from build123d import *

# Parameters (mm, degrees)
CROQUIS1_R              = 2
CROQUIS1_R_2            = 1.5
CROQUIS1_W              = 3
CROQUIS1_H              = 10
SALIENTE_EXTRUIR1_DEPTH = 3


with BuildPart() as part:
    # Croquis1 → Saliente-Extruir1 (new body)
    with BuildSketch(Plane(origin=(0, 0, 0), x_dir=(1, 0, 0), z_dir=(0, 1, 0))):
        with BuildLine():
            Line((-30, -21.975186569), (-30, 62.5))
            Line((-30, 62.5), (-4.123983247, 62.5))
            Line((-4.123983247, 62.5), (-4.123983247, 59.5))
            Line((-4.123983247, 59.5), (5.876016753, 59.5))
            Line((5.876016753, 59.5), (5.876016753, 62.5))
            Line((5.876016753, 62.5), (30, 62.5))
            Line((30, 62.5), (30, -21.975186569))
            Line((30, -21.975186569), (30, -31))
            ThreePointArc((30, -31), (31.171572875, -33.828427125), (34, -35))
            Line((34, -35), (50.699653605, -35))
            ThreePointArc((50.699653605, -35), (55.61862518, -37.564345966), (56.332948449, -43.06542712))
            ThreePointArc((56.332948449, -43.06542712), (44.677053609, -62.460636323), (26.666666667, -76.159540905))
            ThreePointArc((26.666666667, -76.159540905), (20.83772234, -75.883721919), (18, -70.784702406))
            Line((18, -70.784702406), (18, -67.5))
            ThreePointArc((18, -67.5), (16.828427125, -64.671572875), (14, -63.5))
            Line((14, -63.5), (12, -63.5))
            ThreePointArc((12, -63.5), (9.171572875, -64.671572875), (8, -67.5))
            Line((8, -67.5), (8, -80))
            ThreePointArc((8, -80), (0, -88), (-8, -80))
            Line((-8, -80), (-8, -67.5))
            ThreePointArc((-8, -67.5), (-9.171572875, -64.671572875), (-12, -63.5))
            Line((-12, -63.5), (-14, -63.5))
            ThreePointArc((-14, -63.5), (-16.828427125, -64.671572875), (-18, -67.5))
            Line((-18, -67.5), (-18, -70.784702406))
            ThreePointArc((-18, -70.784702406), (-20.83772234, -75.883721919), (-26.666666667, -76.159540905))
            ThreePointArc((-26.666666667, -76.159540905), (-44.677053609, -62.460636323), (-56.332948449, -43.06542712))
            ThreePointArc((-56.332948449, -43.06542712), (-55.61862518, -37.564345966), (-50.699653605, -35))
            Line((-50.699653605, -35), (-34, -35))
            ThreePointArc((-34, -35), (-31.171572875, -33.828427125), (-30, -31))
            Line((-30, -31), (-30, -21.975186569))
        make_face()
        with Locations(Location((-24.3, 37.439181633, 0), (0, 0, 270))):
            Circle(CROQUIS1_R, mode=Mode.SUBTRACT)
        with Locations(Location((16.54, 52.26006939, 0), (0, 0, 270))):
            Circle(CROQUIS1_R_2, mode=Mode.SUBTRACT)
        with Locations(Location((16.54, 34.48006939, 0), (0, 0, 270))):
            Circle(CROQUIS1_R_2, mode=Mode.SUBTRACT)
        with Locations(Location((-16.48, 34.48006939, 0), (0, 0, 270))):
            Circle(CROQUIS1_R_2, mode=Mode.SUBTRACT)
        with Locations(Location((-16.48, 52.26006939, 0), (0, 0, 270))):
            Circle(CROQUIS1_R_2, mode=Mode.SUBTRACT)
        with Locations((28.5, -55)):
            Rectangle(CROQUIS1_W, CROQUIS1_H, mode=Mode.SUBTRACT)
        with Locations((-28.5, -55)):
            Rectangle(CROQUIS1_W, CROQUIS1_H, mode=Mode.SUBTRACT)
        with BuildLine():
            Line((1.5, -65), (1.5, -80))
            ThreePointArc((1.5, -80), (0, -81.5), (-1.5, -80))
            Line((-1.5, -80), (-1.5, -65))
            ThreePointArc((-1.5, -65), (0, -63.5), (1.5, -65))
        make_face(mode=Mode.SUBTRACT)
        with BuildLine():
            Line((7.5, -20), (-7.5, -20))
            ThreePointArc((-7.5, -20), (-11.035533906, -18.535533906), (-12.5, -15))
            Line((-12.5, -15), (-12.5, 15))
            ThreePointArc((-12.5, 15), (-11.035533906, 18.535533906), (-7.5, 20))
            Line((-7.5, 20), (7.5, 20))
            ThreePointArc((7.5, 20), (11.035533906, 18.535533906), (12.5, 15))
            Line((12.5, 15), (12.5, -15))
            ThreePointArc((12.5, -15), (11.035533906, -18.535533906), (7.5, -20))
        make_face(mode=Mode.SUBTRACT)
        with BuildLine():
            ThreePointArc((-52.107977316, -41.51635678), (-41.326274588, -59.456925292), (-24.666666667, -72.12841203))
            ThreePointArc((-24.666666667, -72.12841203), (-22.656290375, -71.451369072), (-23.333333333, -69.440992781))
            ThreePointArc((-23.333333333, -69.440992781), (-39.092421908, -57.454451272), (-49.291329893, -40.48364322))
            ThreePointArc((-49.291329893, -40.48364322), (-51.216010385, -39.591676289), (-52.107977316, -41.51635678))
        make_face(mode=Mode.SUBTRACT)
        with BuildLine():
            ThreePointArc((52.107977316, -41.51635678), (41.326274588, -59.456925292), (24.666666667, -72.12841203))
            ThreePointArc((24.666666667, -72.12841203), (22.656290375, -71.451369072), (23.333333333, -69.440992781))
            ThreePointArc((23.333333333, -69.440992781), (39.092421908, -57.454451272), (49.291329893, -40.48364322))
            ThreePointArc((49.291329893, -40.48364322), (51.216010385, -39.591676289), (52.107977316, -41.51635678))
        make_face(mode=Mode.SUBTRACT)
    extrude(amount=SALIENTE_EXTRUIR1_DEPTH)


solid = part.part
Geometry: final body of the model. Coordinates: model frame, mm. A direction names the side the tool comes from. Coordinates: 2 decimals unless noted, no trailing zeros. Order: outer loops, then holes, each group sorted by start corner. A loop starts at its lowest first (then second) coordinate and runs counter-clockwise, first axis right, second up.
1) Section A-A (x = -44.5). Return loops of the section in (y, z).
Result sheet:
outline: (0, 35) - (3, 35) - (3, 50.27) - (0, 50.27) - close; (0, 55.58) - (3, 55.58) - (3, 62.66) - (0, 62.66) - close
2) Section D-D (x = 36.5). Return loops of the section in (y, z), then the cut area to 3 significant figures.
Result sheet:
outline: (0, 35) - (3, 35) - (3, 60.15) - (0, 60.15) - close; (0, 64.22) - (3, 64.22) - (3, 70.03) - (0, 70.03) - close
area: 92.9 mm2
3) Set-up query: faces 4 (the flat face through (27, 1, 55)), 5 (the flat face through (30, 1, -16)), 6 (the flat face through (1, 1, -59.5)), 7 (the cylindrical face through (16.859, 1.479, 64.703)). Return all of +Z, -Z, +X, -X, +Y, -Y with unobstructed straight access to the full face (end or side cutting, diameter ignored); none if empty.
Result sheet:
face 4: +Y, -Y
face 5: -Z, +X, +Y, -Y
face 6: -Z, +Y, -Y
face 7: +Z, +Y, -Y
4) Ray query, probe 1 along X at (y, z) = (2.45, -2.5); probe 2 along X at (y, z) = (1.05, 57); probe 3 along X at (y, z) = (2.2, 70). Return the intervals inside material, ascending.
Result sheet:
probe 1: x = -30 to -12.5, 12.5 to 30
probe 2: x = -49.03 to -43.4, -39.5 to -30, -27 to 27, 30 to 39.5, 43.4 to 49.03
probe 3: x = -36.54 to -28.56, -22.72 to -18, -8 to -1.5, 1.5 to 8, 18 to 22.72, 28.56 to 36.54
5) Section B-B (z = 74). Return loops of the section in (x, y).
Result sheet:
outline: (-30.64, 0) - (-18.93, 0) - (-18.93, 3) - (-30.64, 3) - close; (-8, 0) - (-1.5, 0) - (-1.5, 3) - (-8, 3) - close; (1.5, 0) - (8, 0) - (8, 3) - (1.5, 3) - close; (18.93, 0) - (30.64, 0) - (30.64, 3) - (18.93, 3) - close
6) Section C-C (y = 0.75). Give the number of separate pieces and of enclosed holes in the cut face, then the cut area to 3 significant figures.
Result sheet:
separate pieces: 1
enclosed holes: 11
area: 8,250 mm2
7) Draft query along Z for faces 1 (the cylindrical face through (-44.46, 1.48, 62.7)), 2 (the flat face through (-4.124, 1, -61)), 3 (the cylindrical face through (-17.81, 1.48, -51.57)). Return one class per face: released by +Z, released by -Z, zero draft, split by the parting line, or undercut.
Result sheet:
face 1: released by +Z
face 2: zero draft
face 3: undercut
8) First-contact query: P1, Ø1.5, axis at y = 1, z = 66.5, coming from the -X side; P2, Ø0.9, axis at x = 0.5, y = 1, coming from the -Z side; P3, Ø1.5, axis at x = 36, y = 1.5, coming from the +Z side. Flat tips, straight axial feed; report the tip coordinate or a pass-through.
Result sheet:
P1: stops at x = -41.49
P2: stops at z = -59.5
P3: stops at z = 70.96
